Source: CAD feature listing. Evaluate the final solid. Frame: model axes, mm. Face numbers are marked on the shaded views. Coordinates: 2 decimals unless noted, no trailing zeros.
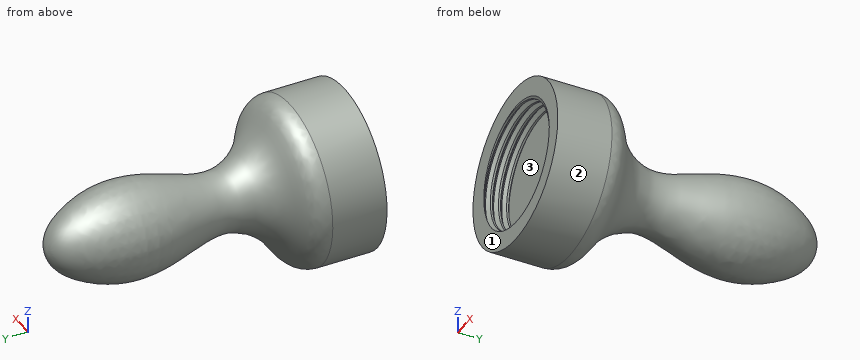
```python
from build123d import *

# Parameters (mm, degrees)
ROSCA1_PITCH          = 1.5
CORTAR_EXTRUIR1_START = 10
CROQUIS3_R            = 15
CORTAR_EXTRUIR1_DEPTH = 10


with BuildPart() as part:
    # Croquis1 → Revolución1 (revolve)
    with BuildSketch(Plane.XY, mode=Mode.PRIVATE) as revoluci_n1_sk:
        with BuildLine():
            Line((-12, 0), (-12, 5))
            Line((-12, 5), (0, 5))
            Line((0, 5), (0, 55))
            add(Edge.make_bspline(
                [(0, 55), (-3.180764289, 54.869157284), (-6.802128833, 49.987752556), (-9.296892214, 41.327039564), (-7.460278375, 32.164910722), (-3.920844043, 22.793687376), (-9.40714477, 14.872769973), (-14.838813261, 12.976020169), (-15, 10)],
                knots=[0, 0, 0, 0, 0.153337628, 0.314153231, 0.514828567, 0.684692443, 0.859563088, 1, 1, 1, 1], degree=3))
            Line((-15, 10), (-15, 0))
            Line((-15, 0), (-12, 0))
        make_face()
    revolve(revoluci_n1_sk.sketch.rotate(Axis((0, 5, 0), (0, 1, 0)), 270), axis=Axis((0, 5, 0), (0, 1, 0)))

    # Rosca1: the profile of Perfil de rosca1 profile screwed along a right-hand helix of 4.333333 turns, 8 arcs to a turn; built about Z, then put on its axis
    rosca1_z = Axis((0, 0, 0), (0, 0, 1))
    rosca1_corners = [(12.0003, 0, -0.000173205), (12.0003, 0, 1.312673201), (11.188101187, 0, 0.843749998), (11.188101187, 0, 0.468749998)]
    with BuildLine(mode=Mode.PRIVATE) as rosca1_profile:
        Line(rosca1_corners[0], rosca1_corners[1])
        Line(rosca1_corners[1], rosca1_corners[2])
        Line(rosca1_corners[2], rosca1_corners[3])
        Line(rosca1_corners[3], rosca1_corners[0])
    rosca1_cap = Face(rosca1_profile.wire())
    rosca1_turn_angles = [0, 22.5, 45, 67.5, 90, 112.5, 135, 157.5, 180, 202.5, 225, 247.5, 270, 292.5, 315, 337.5, 360]
    rosca1_turn_weights = [1, 0.9238795325112867, 1, 0.9238795325112867, 1, 0.9238795325112867, 1, 0.9238795325112867, 1, 0.9238795325112867, 1, 0.9238795325112867, 1, 0.9238795325112867, 1, 0.9238795325112867, 1]
    rosca1_turn_rails = [Edge.make_bspline([Vector(p[0], p[1], 0).rotate(rosca1_z, rosca1_turn_angles[k]) / rosca1_turn_weights[k] + Vector(0, 0, p[2] + ROSCA1_PITCH * rosca1_turn_angles[k] / 360) for k in range(17)], [0, 0, 0, 1, 1, 2, 2, 3, 3, 4, 4, 5, 5, 6, 6, 7, 7, 8, 8, 8], 2, rosca1_turn_weights) for p in rosca1_corners]
    rosca1_turn_sides = [Face.make_surface_from_curves(rosca1_turn_rails[p[0]], rosca1_turn_rails[p[1]]) for p in [(0, 1), (1, 2), (2, 3), (3, 0)]]
    rosca1_last_angles = [1440, 1462.5, 1485, 1507.5, 1530, 1545, 1560]
    rosca1_last_weights = [1, 0.9238795325112867, 1, 0.9238795325112867, 1, 0.9659258262890683, 1]
    rosca1_last_rails = [Edge.make_bspline([Vector(p[0], p[1], 0).rotate(rosca1_z, rosca1_last_angles[k]) / rosca1_last_weights[k] + Vector(0, 0, p[2] + ROSCA1_PITCH * rosca1_last_angles[k] / 360) for k in range(7)], [0, 0, 0, 1, 1, 2, 2, 3, 3, 3], 2, rosca1_last_weights) for p in rosca1_corners]
    rosca1_last_sides = [Face.make_surface_from_curves(rosca1_last_rails[p[0]], rosca1_last_rails[p[1]]) for p in [(0, 1), (1, 2), (2, 3), (3, 0)]]
    rosca1 = Plane(origin=(0, -1.5, 0), x_dir=(1, 0, 0), z_dir=(0, 1, 0)) * Solid(Shell([*[p.moved(Location((0, 0, ROSCA1_PITCH * i))) for i in range(4) for p in rosca1_turn_sides], *rosca1_last_sides, rosca1_cap, rosca1_cap.rotate(rosca1_z, 1560).moved(Location((0, 0, ROSCA1_PITCH * 1560 / 360)))]))
    add(rosca1)

    # Croquis3 → Cortar-Extruir1 (cut)
    with BuildSketch(Plane.XZ.offset(CORTAR_EXTRUIR1_START)):
        with Locations(Location((0, 0, 0), (0, 0, 270))):
            Circle(CROQUIS3_R)
    extrude(amount=-CORTAR_EXTRUIR1_DEPTH, mode=Mode.SUBTRACT)


solid = part.part
```
Q1. Material intervals for line 1 along Z through (x, y) = (0, 1); line 2 along Z through (x, y) = (0, 2); line 3 along Y through (x, z) = (-5, 5), sorted ascending.
Q2. Draft query along Z for the marked faces 1, 2 and 3. Return one class per face: released by +Z, released by -Z, zero draft, split by the parting line, or undercut.
Q3. First-contact query: pin 1 Ø6 at (y, z) = (42, 3) entering from +X; pin 2 Ø5 at (y, z) = (35.5, -1.5) entering from +X; pin 3 Ø4 at (y, z) = (38.5, 3.5) entering from -X. Flat tips, straight axial feed; report the tip coordinate or a pass-through.
Resolved:
1. line 1: z = -15 to -11.19, 12 to 15
1. line 2: z = -15 to -11.78, 11.24 to 15
1. line 3: y = 5 to 18.77, 31.8 to 48.13
2. face 1: zero draft
2. face 2: split by the parting line
2. face 3: undercut
3. pin 1: stops at x = 8.55
3. pin 2: stops at x = 8.36
3. pin 3: stops at x = -8.35
